from build123d import *

# Parameters (mm, degrees)
SKETCH_1_W          = 49
SKETCH_1_H          = 64
EXTRUDE_1_DEPTH     = 3
SKETCH_2_W          = 5
SKETCH_2_H          = 64
EXTRUDE_2_DEPTH     = 4
SKETCH_3_R          = 1.15
CUT_EXTRUDE_2_DEPTH = 69.645830172
FILLET_1_R          = 2.5
FILLET_2_R          = 4
CUT_EXTRUDE_3_DEPTH = 1.2


with BuildPart() as part:
    # 草图1 → 凸台-拉伸1 (new body)
    with BuildSketch(Plane(origin=(0, 0, 0), x_dir=(1, 0, 0), z_dir=(0, 1, 0))):
        Rectangle(SKETCH_1_W, SKETCH_1_H)
    extrude(amount=EXTRUDE_1_DEPTH)

    # 草图2 → 凸台-拉伸2 (add)
    with BuildSketch(Plane(origin=(0, 0, 0), x_dir=(-1, 0, 0), z_dir=(0, -1, 0))):
        with Locations((-22, 0)):
            Rectangle(SKETCH_2_W, SKETCH_2_H)
    extrude(amount=EXTRUDE_2_DEPTH)

    # 草图3 → 切除-拉伸2 (cut, through all)
    with BuildSketch(Plane(origin=(0, 0, -32), x_dir=(-1, 0, 0), z_dir=(0, 0, -1))):
        with Locations((-22, -1.3)):
            Circle(SKETCH_3_R)
    extrude(amount=-CUT_EXTRUDE_2_DEPTH, mode=Mode.SUBTRACT)

    # 圆角1
    fillet_1_edges = [part.edges().sort_by_distance(p)[0] for p in [
        (24.5, -4, 0),
        (19.5, -4, 0),
    ]]
    fillet(fillet_1_edges, radius=FILLET_1_R - 0.0001)  # a hair under: the kernel refuses the full size

    # 圆角2
    fillet_2_edges = [part.edges().sort_by_distance(p)[0] for p in [
        (24.5, 3, 0),
    ]]
    fillet(fillet_2_edges, radius=FILLET_2_R)

    # 草图4 → 切除-拉伸3 (cut)
    with BuildSketch(Plane(origin=(0, 0, 0), x_dir=(-1, 0, 0), z_dir=(0, -1, 0))):
        with BuildLine():
            Line((24.5, -28), (24.5, -32))
            Line((24.5, -32), (20.5, -32))
            ThreePointArc((20.5, -32), (21.671572875, -29.171572875), (24.5, -28))
        make_face()
        with BuildLine():
            Line((24.5, 28), (24.5, 32))
            Line((24.5, 32), (20.5, 32))
            ThreePointArc((20.5, 32), (21.671572875, 29.171572875), (24.5, 28))
        make_face()
    extrude(amount=-CUT_EXTRUDE_3_DEPTH, mode=Mode.SUBTRACT)


solid = part.part
Geometry check sheet. Reference: the model listing, model coordinates, mm. A direction names the side the tool comes from. Give positions to 0.01 mm unless a question says otherwise; leave off trailing zeros. Loops run counter-clockwise (first coordinate to the right, second up) from the corner with the lowest first, then second, coordinate; pieces in that order, holes last.
(1) Section check C-C on y = 2. Record the cut outline in (x, z).
From the geometry:
outline: (-24.5, -32) - (23.15, -32) - (23.15, 32) - (-24.5, 32) - close
(2) Release check for a two-part mould opening along Y. For faces 1 (the cylindrical face through (24, -3, 0)), 2 (the flat face through (0, 1, 32)), 3 (the cylindrical face through (22.848, -0.523, -0.448)), 4 (the flat face through (-2, 3, 0)) record: released by +Y, released by -Y, zero draft, split by the parting line, or undercut.
From the geometry:
face 1: released by -Y
face 2: zero draft
face 3: undercut
face 4: released by +Y
(3) Set-up check for faces 5 (the cylindrical face through (-21.641, 0.592, 29.203)), 6 (the flat face through (-3, 0, 0)), 7 (the flat face through (-23, 1.2, -30)): record each of +Z, -Z, +X, -X, +Y, -Y from which the full face is reachable in a straight line by a thin tool's end or side.
From the geometry:
face 5: +Z, -X, -Y
face 6: +Z, -Z, -X, -Y
face 7: -Z, -X, -Y
(4) Section check B-B on x = -18. Record the cut outline in (y, z).
From the geometry:
outline: (0, -32) - (3, -32) - (3, 32) - (0, 32) - close
(5) Depth check by flat-ended pin: pin 1 Ø4.5 at (x, z) = (-21.5, 30) entering from -Y; pin 2 Ø1.4 at (x, y) = (22, -1.3) entering from +Z; pin 3 Ø1.2 at (y, z) = (-0.5, 14.5) entering from -X. Enter the tip coordinate at first touch or a pass-through.
From the geometry:
pin 1: stops at y = 0
pin 2: passes through
pin 3: stops at x = -24.5
(6) Thickness scan on L1, parallel to Y at x = -1, z = -24; L2, parallel to Y at x = 22, z = 2.5; L3, parallel to X at y = -0.25, z = -19.5. Record the ranges inside material, lowest first.
From the geometry:
L1: y = 0 to 3
L2: y = -4 to -2.45, -0.15 to 2.71
L3: x = 19.5 to 21.53, 22.47 to 24.43
